from build123d import *

# Parameters (mm, degrees)
SKETCH5_R           = 2.525
SKETCH5_R_2         = 3.025
BOSS_EXTRUDE2_DEPTH = 15.748
SKETCH6_W           = 11
SKETCH6_H           = 12.1
CUT_EXTRUDE2_DEPTH  = 12.7


with BuildPart() as part:
    # Sketch5 → Boss-Extrude2 (new body, symmetric)
    with BuildSketch(Plane.XY):
        with BuildLine():
            Line((-20.6375, 4.7625), (20.6375, 4.7625))
            ThreePointArc((20.6375, 4.7625), (25.4, 0), (20.6375, -4.7625))
            Line((20.6375, -4.7625), (-20.6375, -4.7625))
            ThreePointArc((-20.6375, -4.7625), (-25.4, 0), (-20.6375, 4.7625))
        make_face()
        with Locations((-20.6375, 0)):
            Circle(SKETCH5_R, mode=Mode.SUBTRACT)
        with Locations((20.6375, 0)):
            Circle(SKETCH5_R_2, mode=Mode.SUBTRACT)
    extrude(amount=BOSS_EXTRUDE2_DEPTH, both=True)

    # Sketch6 → Cut-Extrude2 (cut, symmetric)
    with BuildSketch(Plane(origin=(0, 0, 0), x_dir=(1, 0, 0), z_dir=(0, 1, 0))):
        with Locations((-19.9, 6.698)):
            Rectangle(SKETCH6_W, SKETCH6_H)
    extrude(amount=CUT_EXTRUDE2_DEPTH, both=True, mode=Mode.SUBTRACT)


solid = part.part
Check sheet for the modelled part. Datum: model origin and axes. Units: mm. A direction names the side the tool comes from. Give positions to 0.01 mm unless a question says otherwise; leave off trailing zeros. Write each loop counter-clockwise with the first axis right and the second up, starting at its lowest first coordinate (ties: lowest second). Pieces come first, ordered by that corner, then holes. Notation, with made-up numbers: (68, 37.5) -> (79, 37.5) arc R20 cw to (79, 51.5) -> close; hole circle Ø9 at (65.25, 84). An arc over 180 degrees is marked (long way). Write item = value, one per line.
Item 1: Sectioned sample at B-B on y = 0. Record the boundary of the cut face in (x, z).
Output:
outline = (-25.4, -15.75) -> (-23.16, -15.75) -> (-23.16, -12.75) -> (-25.4, -12.75) -> close; (-25.4, -0.65) -> (-23.16, -0.65) -> (-23.16, 15.75) -> (-25.4, 15.75) -> close; (-18.11, -15.75) -> (17.61, -15.75) -> (17.61, 15.75) -> (-18.11, 15.75) -> (-18.11, -0.65) -> (-14.4, -0.65) -> (-14.4, -12.75) -> (-18.11, -12.75) -> close; (23.66, -15.75) -> (25.4, -15.75) -> (25.4, 15.75) -> (23.66, 15.75) -> close
Item 2: Tool access check on faces 5 (the cylindrical face through (-23.16, 0.11, 7.44)), 6 (the flat face through (-17.5, 0.1, -0.648)). Record the directions out of +Z, -Z, +X, -X, +Y, -Y that give a thin tool (end or side, any length) a straight path to the whole face; none if there is none.
Output:
face_5 = +Z, -Z
face_6 = -X, +Y, -Y
Item 3: Scan lines: probe 1 along Z at (x, y) = (-18.5, 1.5); probe 2 along X at (y, z) = (0.5, 6); probe 3 along X at (y, z) = (-2.25, -0.5). Record each from-to range of solid material in increasing order. Write a range as from..to.
Output:
probe_1 = -15.75..-12.75, -0.65..15.75
probe_2 = -25.37..-23.11, -18.16..17.65, 23.62..25.37
probe_3 = -24.83..-21.78, -19.49..18.62, 22.66..24.83
Item 4: Sectioned sample at A-A on x = -16. Record the boundary of the cut face in (y, z), and give its area (3 significant figures).
Output:
outline = (-4.76, -15.75) -> (4.76, -15.75) -> (4.76, -12.75) -> (-4.76, -12.75) -> close; (-4.76, -0.65) -> (4.76, -0.65) -> (4.76, 15.75) -> (-4.76, 15.75) -> close
area = 185 mm^2
Item 5: Gauge pin test, flat ends, axial feed: pin 1 (3 mm diameter, centred on y = 0, z = -6.5, fed in from -X); pin 2 (3 mm diameter, centred on x = -20.64, y = 0, fed in from -Z); pin 3 (1 mm diameter, centred on y = -2.5, z = -1.5, fed in from +X); pin 4 (3 mm diameter, centred on x = -21.5, y = -1.5, fed in from -Z). Record the tip position at first contact, or that the pin passes through.
Output:
pin_1 = -14.4
pin_2 = through
pin_3 = 24.96
pin_4 = -15.75
Item 6: Release check for a two-part mould opening along Z. For faces 1 (the flat face through (-14.4, 0, -7)), 2 (the cylindrical face through (-23.16, 0.11, -14.27)), 3 (the flat face through (0, 0, -15.748)), 4 (the flat face through (-17.5, 0.1, -12.748)) record: +Z half, -Z half, draft (parallel to the pull), parting line (faces both ways), or undercut.
Output:
face_1 = undercut
face_2 = draft
face_3 = -Z half
face_4 = undercut
